Input: part model. Units: mm. Frame: model coordinates. Face numbers are marked on the shaded views. A direction names the side the tool comes from. Coordinates: 2 decimals unless noted, no trailing zeros. Order: outer loops, then holes, each group sorted by start corner. A loop starts at its lowest first (then second) coordinate and runs counter-clockwise, first axis right, second up. Notation, with made-up numbers: (61, 47) - (81, 47) arc R20 ccw to (81, 64) - close; hole circle Ø9 at (21.5, -13.75). An arc over 180 degrees is marked (long way). One line per question, with ' | ' between items.
from build123d import *

# Parameters (mm, degrees)
EXTRUDE_1_DEPTH = 2.9
SKETCH_2_R      = 1.25
EXTRUDE_2_DEPTH = 1.5
FILLET_1_R      = 5
FILLET_2_R      = 0.5


with BuildPart() as part:
    # 草图1 → 凸台-拉伸1 (new body)
    with BuildSketch(Plane.XY):
        with BuildLine():
            Line((-7.635161831, 28.494811876), (-6.729295173, 25.114071484))
            ThreePointArc((-6.729295173, 25.114071484), (0, 26), (6.729295173, 25.114071484))
            Line((6.729295173, 25.114071484), (7.635161831, 28.494811876))
            ThreePointArc((7.635161831, 28.494811876), (0, 29.5), (-7.635161831, 28.494811876))
        make_face()
    extrude(amount=EXTRUDE_1_DEPTH)

    # 草图2 → 凸台-拉伸2 (add)
    with BuildSketch(Plane.XY.offset(2.9)):
        with BuildLine():
            Line((-7.635161831, 28.494811876), (-4.658742812, 17.386664873))
            ThreePointArc((-4.658742812, 17.386664873), (0, 18), (4.658742812, 17.386664873))
            Line((4.658742812, 17.386664873), (7.635161831, 28.494811876))
            ThreePointArc((7.635161831, 28.494811876), (0, 29.5), (-7.635161831, 28.494811876))
        make_face()
        with Locations((0, 22.5)):
            Circle(SKETCH_2_R, mode=Mode.SUBTRACT)
    extrude(amount=EXTRUDE_2_DEPTH)

    # 圆角1
    fillet_1_edges = [part.edges().sort_by_distance(p)[0] for p in [
        (-4.658742812, 17.386664873, 3.65),
        (4.658742812, 17.386664873, 3.65),
    ]]
    fillet(fillet_1_edges, radius=FILLET_1_R)

    # 圆角2
    fillet_2_edges = [part.edges().sort_by_distance(p)[0] for p in [
        (0, 26, 0),
    ]]
    fillet(fillet_2_edges, radius=FILLET_2_R)


solid = part.part
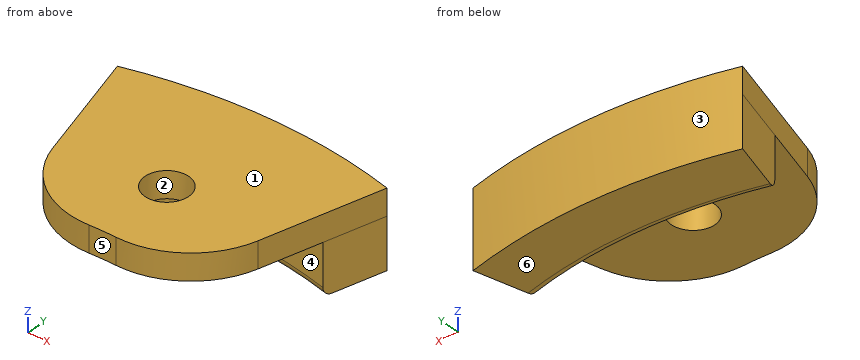
Item 1: Contact query for flat-ended pins moving along their axis: P1, Ø1, axis at y = 27.5, z = 1, coming from the +X side; P2, Ø1.5, axis at x = 3.5, y = 19.5, coming from the -Z side. Output: stop coordinate, or through.
Data:
P1: x = 7.5 | P2: z = 2.9
Item 2: Access query for the marked faces 4, 5 and 6. Directions: +Z, -Z, +X, -X, +Y, -Y. A direction counts if a zero-diameter tool reaches every point of the face in a straight line with its end or side. Return the directions, or none.
Data:
face 4: -Z, -Y | face 5: +Z, -Z, -Y | face 6: -Z, +X, -X, +Y, -Y
Item 3: Section D-D on z = 1.7. Return the cut outline in (x, y).
Data:
outline: (-7.64, 28.49) - (-6.73, 25.11) arc R26 cw to (6.73, 25.11) - (7.64, 28.49) arc R29.5 ccw to start
Item 4: Section A-A on x = 0. Return the cut outline in (y, z).
Data:
outline: (18, 2.9) - (21.25, 2.9) - (21.25, 4.4) - (18, 4.4) - close; (23.75, 2.9) - (26, 2.9) - (26, 0.5) arc R0.5 ccw to (26.5, 0) - (29.5, 0) - (29.5, 4.4) - (23.75, 4.4) - close
Item 5: Section B-B on z = 3.55. Return the cut outline in (x, y).
Data:
outline: (-7.64, 28.49) - (-5.81, 21.68) arc R5 ccw to (-0.77, 17.98) arc R18 cw to (0.77, 17.98) arc R5 ccw to (5.81, 21.68) - (7.64, 28.49) arc R29.5 ccw to start; hole circle Ø2.5 at (0, 22.5)
Item 6: Section C-C on y = 22.5. Return the cut outline in (x, z).
Data:
outline: (-6.03, 2.9) - (-1.25, 2.9) - (-1.25, 4.4) - (-6.03, 4.4) - close; (1.25, 2.9) - (6.03, 2.9) - (6.03, 4.4) - (1.25, 4.4) - close
Item 7: Ray query, line 1 (Z direction, x = 0, y = 25.5); line 2 (Y direction, x = 0, z = 3.95); line 3 (X direction, y = 21.75, z = 3.2). Return the intervals inside material, ascending.
Data:
line 1: 2.9 to 4.4 | line 2: 18 to 21.25, 23.75 to 29.5 | line 3: -5.83 to -1, 1 to 5.83
Item 8: Draft query along X for the marked faces 1, 2 and 3. Return one class per face: released by +X, released by -X, zero draft, split by the parting line, or undercut.
Data:
face 1: zero draft | face 2: undercut | face 3: split by the parting line
